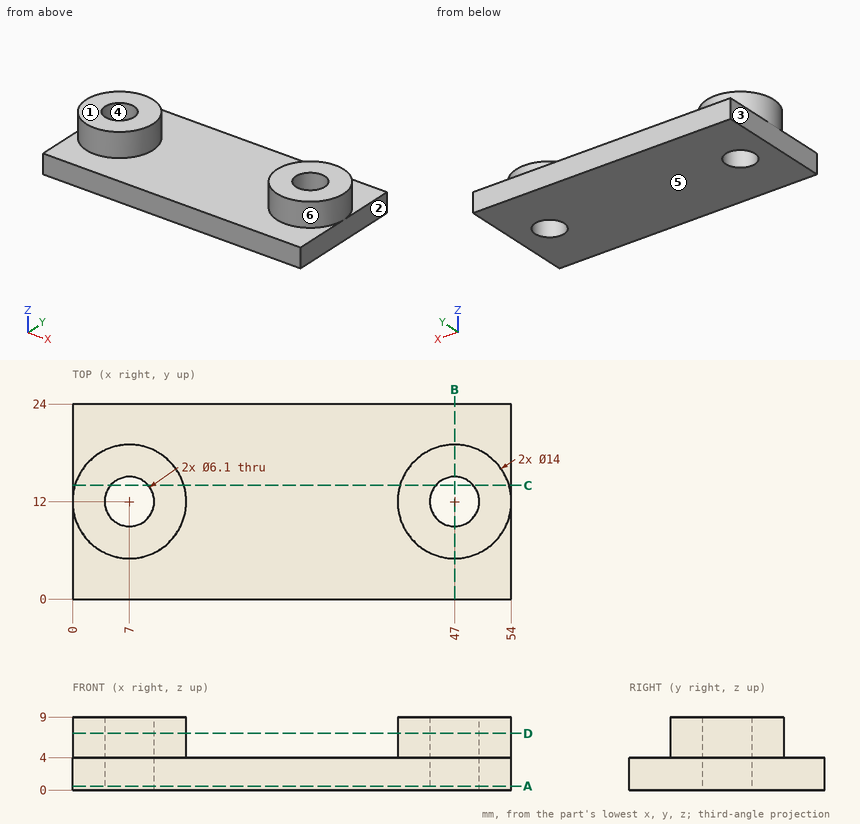
Geometry: see drawing. Coordinates: mm, zero at the bounding-box minimum. A direction names the side the tool comes from. Round coordinates to 2 decimals unless told otherwise and drop trailing zeros. Loops run counter-clockwise (first coordinate to the right, second up) from the corner with the lowest first, then second, coordinate; pieces in that order, holes last. Notation, with made-up numbers: (84.5, 33) -> (93.5, 33) arc R12 cw to (93.5, 38) -> close; hole circle Ø8 at (46.25, 44.25). An arc over 180 degrees is marked (long way). Write each question's results on one line, items separated by ' | '.
Item 1: Pin query (flat end, axial travel): pin 1 Ø5 at (x, z) = (44, 7.5) entering from -Y; pin 2 Ø5.5 at (x, y) = (7, 12) entering from -Z. Return the tip coordinate at first contact, or that it passes through.
Answers below:
pin 1: stops at y = 5.02 | pin 2: passes through
Item 2: Cut plane A-A on z = 0.5. Return the cut outline in (x, y).
Answers below:
outline: (0, 0) -> (54, 0) -> (54, 24) -> (0, 24) -> close; hole circle Ø6.1 at (7, 12); hole circle Ø6.1 at (47, 12)
Item 3: Cut plane D-D on z = 7. Return the cut outline in (x, y), and give its area (3 significant figures).
Answers below:
outline: circle Ø14 at (7, 12); circle Ø14 at (47, 12); hole circle Ø6.1 at (7, 12); hole circle Ø6.1 at (47, 12) | area: 249 mm²
Item 4: Pull-direction query (X, two-part tool) for the marked faces 1, 2, 3 and 4; classes: pulls with the +X half, pulls with the -X half, needs draft (parallel to the pull), parting line crosses it, or undercut.
Answers below:
face 1: needs draft | face 2: pulls with the +X half | face 3: pulls with the -X half | face 4: undercut
Item 5: Cut plane C-C on y = 14. Return the cut outline in (x, z), and give its area (3 significant figures).
Answers below:
outline: (0, 0) -> (4.7, 0) -> (4.7, 9) -> (0.29, 9) -> (0.29, 4) -> (0, 4) -> close; (9.3, 0) -> (44.7, 0) -> (44.7, 9) -> (40.29, 9) -> (40.29, 4) -> (13.71, 4) -> (13.71, 9) -> (9.3, 9) -> close; (49.3, 0) -> (54, 0) -> (54, 4) -> (53.71, 4) -> (53.71, 9) -> (49.3, 9) -> close | area: 267 mm²
Item 6: Set-up query: the marked faces 5 and 6. Return all of +Z, -Z, +X, -X, +Y, -Y with unobstructed straight access to the full face (end or side cutting, diameter ignored); none if empty.
Answers below:
face 5: -Z, +X, -X, +Y, -Y | face 6: +Z
Item 7: Cut plane B-B on x = 47. Return the cut outline in (y, z).
Answers below:
outline: (0, 0) -> (8.95, 0) -> (8.95, 9) -> (5, 9) -> (5, 4) -> (0, 4) -> close; (15.05, 0) -> (24, 0) -> (24, 4) -> (19, 4) -> (19, 9) -> (15.05, 9) -> close
Item 8: Line query: probe 1 along Z at (x, y) = (24.5, 9.5); probe 2 along X at (y, z) = (5.75, 6); probe 3 along X at (y, z) = (6.25, 4.5). Output: solid intervals per line, ascending. Write a range as [from, to].
Answers below:
probe 1: z = [0, 4] | probe 2: x = [3.85, 10.15], [43.85, 50.15] | probe 3: x = [3.01, 10.99], [43.01, 50.99]
